Could you check a few things on this model? Use its own coordinates, in mm. Give positions to 0.01 mm unless a question says otherwise; leave off trailing zeros. Order: outer loops, then holes, each group sorted by start corner. A loop starts at its lowest first (then second) coordinate and runs counter-clockwise, first axis right, second up.
(1) If I drill on probe 1 along X at (y, z) = (2.35, -29.5), over which ranges is the centre line in solid material (lowest first)?
(2) Imagine slicing it at A-A, the plane z = 19. Write out the boundary of the cut face in (x, y).
(3) Will these pins go through, and if not, where does the flat tip stop? pin 1 (1.4 mm diameter, centred on x = -44.5, z = 1, fed in from -Y); pin 2 (0.6 mm diameter, centred on y = 2.5, z = -12, fed in from -X); pin 3 (0.9 mm diameter, centred on x = -45.5, z = 21.5, fed in from +Y).
from build123d import *

# Parameters (mm, degrees)
F0_W     = 43.6125099659
F0_H     = 91.5184393525
F1_DEPTH = 2.5
F2_W     = 0.9
F2_H     = 91.5184393525
F3_DEPTH = 2.9


# Not quite as in the source:
# - a feature of the source that left no trace in its solid (it failed there, or was rolled back) is left out


with BuildPart() as f1:
    # F0 (on Front) → F1 (new body)
    with BuildSketch(Plane.XZ):
        with Locations((-21.8062549829, 0)):
            Rectangle(F0_W, F0_H)
    extrude(amount=-F1_DEPTH)

    # F2 (on face) → F3 (join)
    with BuildSketch(Plane(origin=(-43.6125099659, 0, 0), x_dir=(0, -1, 0), z_dir=(-1, 0, 0))):
        with Locations((-1.25, 0)):
            Rectangle(F2_W, F2_H)
    extrude(amount=F3_DEPTH)


solid = f1.part
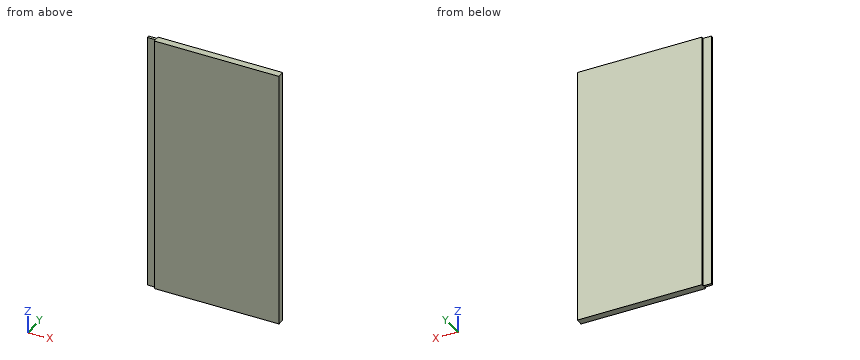
Answer block:
1. probe 1: x = -43.61 to 0
2. outline: (-46.51, 0.8) - (-43.61, 0.8) - (-43.61, 0) - (0, 0) - (0, 2.5) - (-43.61, 2.5) - (-43.61, 1.7) - (-46.51, 1.7) - close
3. pin 1: stops at y = 0.8
3. pin 2: stops at x = -43.61
3. pin 3: stops at y = 1.7
